Autodesk Inventor part; units mm, degrees
ref_plane "YZ Plane" through (0, 0, 0) normal (1, 0, 0) x (0, 1, 0)
ref_plane "XZ Plane" through (0, 0, 0) normal (0, 1, 0) x (-1, 0, 0)
ref_plane "XY Plane" through (0, 0, 0) normal (0, 0, 1) x (1, 0, 0)
sketch "Sketch1" plane through (0, 0, 0) normal (0, 0, 1) x (1, 0, 0)
  line L0 (0, 0) -> (90, 0)
  line L1 (90, 0) -> (90, -160)
  line L2 (90, -160) -> (0, -160)
  line L3 (0, -160) -> (0, 0)
  dimension "d0" = 90
  dimension "d1" = 160
extrude "Extrusion1" add sketch "Sketch1" along normal blind 1.6
sketch "Sketch2" plane through (0, 0, 1.6) normal (0, 0, 1) x (1, 0, 0)
  line L0 (5, -5) -> (85, -5)
  line L1 (85, -5) -> (85, -15)
  line L2 (85, -15) -> (5, -15)
  line L3 (5, -15) -> (5, -5)
  line L4 (90, 0) -> (0, 0)
  line L5 (0, 0) -> (0, -160)
  line L6 (90, -160) -> (90, 0)
  line L7 (5, -5) -> (15, -5)
  line L8 (15, -5) -> (15, -155)
  line L9 (15, -155) -> (5, -155)
  line L10 (5, -155) -> (5, -5)
  line L11 (0, -160) -> (90, -160)
  line L12 (5, -155) -> (85, -155)
  line L13 (85, -155) -> (85, -145)
  line L14 (85, -145) -> (5, -145)
  line L15 (5, -145) -> (5, -155)
  line L16 (85, -5) -> (75, -5)
  line L17 (75, -5) -> (75, -155)
  line L18 (75, -155) -> (85, -155)
  line L19 (85, -155) -> (85, -5)
  line L20 (5, -75) -> (85, -75)
  line L21 (85, -75) -> (85, -85)
  line L22 (85, -85) -> (5, -85)
  line L23 (5, -85) -> (5, -75)
  dimension "d4" = 5
  dimension "d5" = 5
  dimension "d6" = 5
  dimension "d7" = 10
  dimension "d8" = 10
  dimension "d9" = 5
  dimension "d10" = 80
  dimension "d11" = 10
  dimension "d12" = 10
  dimension "d13" = 80
  dimension "d14" = 10
  dimension "d15" = 75
extrude "Extrusion2" add sketch "Sketch2" along normal blind 4.6 contours L0 L8 L2 L3 | L0 L17 L2 L8 | L2 L8 L20 L10 | L0 L1 L2 L17 | L20 L8 L22 L10 | L2 L19 L20 L17 | L20 L17 L22 L8 | L22 L8 L14 L10 | L20 L19 L22 L17 | L14 L8 L9 L10 | L22 L19 L14 L17 | L14 L17 L12 L8 | L14 L13 L12 L17
sketch "Sketch3" plane through (0, 0, 6.2) normal (0, 0, 1) x (1, 0, 0)
  circle A0 centre (20, -10) radius 2.6
  circle A1 centre (53.3333, -10) radius 2.6
  circle A2 centre (36.6667, -10) radius 2.6
  circle A3 centre (80, -140) radius 2.6
  circle A4 centre (80, -123.3333) radius 2.6
  circle A5 centre (80, -107) radius 2.6
  circle A6 centre (80, -90) radius 2.6
  circle A7 centre (70, -150) radius 2.6
  circle A8 centre (53.3333, -150) radius 2.6
  circle A9 centre (36.6667, -150) radius 2.6
  circle A10 centre (20, -150) radius 2.6
  circle A11 centre (10, -140) radius 2.6
  circle A12 centre (10, -123.3333) radius 2.6
  circle A13 centre (10, -106.6667) radius 2.6
  circle A14 centre (10, -90) radius 2.6
  circle A15 centre (70, -80) radius 2.6
  circle A16 centre (53.3333, -80) radius 2.6
  circle A17 centre (36.6667, -80) radius 2.6
  circle A18 centre (20, -80) radius 2.6
  circle A19 centre (80, -70) radius 2.6
  circle A20 centre (80, -53.3333) radius 2.6
  circle A21 centre (80, -36.6667) radius 2.6
  circle A22 centre (80, -20) radius 2.6
  circle A23 centre (10, -70) radius 2.6
  circle A24 centre (10, -53.3333) radius 2.6
  circle A25 centre (10, -36.6667) radius 2.6
  circle A26 centre (10, -20) radius 2.6
  circle A27 centre (70, -10) radius 2.6
  line L0 (85, -155) -> (5, -155)
  line L1 (85, -5) -> (5, -5)
  line L2 (5, -5) -> (5, -155)
  line L3 (15, -75) -> (15, -15)
  line L4 (75, -15) -> (75, -75)
  line L5 (15, -15) -> (75, -15)
  line L6 (85, -155) -> (85, -5)
  line L7 (15, -85) -> (75, -85)
  line L8 (15, -145) -> (15, -85)
  point P0 (0, 0)
  point P1 (90, -155)
  dimension "d18" = 5.2
  dimension "d20" = 5.2
  dimension "d21" = 5.2
  dimension "d22" = 5.2
  dimension "d23" = 5.2
  dimension "d24" = 5.2
  dimension "d25" = 5.2
  dimension "d26" = 5.2
  dimension "d27" = 5.2
  dimension "d28" = 5.2
  dimension "d29" = 5.2
  dimension "d30" = 5.2
  dimension "d31" = 5.2
  dimension "d32" = 5.2
  dimension "d33" = 5.2
  dimension "d34" = 5.2
  dimension "d35" = 5.2
  dimension "d36" = 5.2
  dimension "d37" = 5.2
  dimension "d38" = 5.2
  dimension "d39" = 5.2
  dimension "d40" = 5.2
  dimension "d41" = 5.2
  dimension "d42" = 5.2
  dimension "d43" = 5.2
  dimension "d44" = 5.2
  dimension "d45" = 5.2
  dimension "d47" = 5.2
  dimension "d48" = 5
  dimension "d49" = 5
  dimension "d50" = 5
  dimension "d51" = 5
  dimension "d52" = 5
  dimension "d53" = 5
  dimension "d55" = 5
  dimension "d56" = 16.6667
  dimension "d57" = 16.6667
  dimension "d58" = 5
  dimension "d59" = 16.6667
  dimension "d60" = 16.6667
  dimension "d61" = 16.6667
  dimension "d62" = 5
  dimension "d63" = 5
  dimension "d64" = 5
  dimension "d65" = 16.6667
  dimension "d66" = 16.6667
  dimension "d67" = 16.6667
  dimension "d68" = 5
  dimension "d73" = 16.6667
  dimension "d74" = 16.6667
  dimension "d75" = 16.6667
extrude "Extrusion3" cut sketch "Sketch3" against normal through all contours A0 | A1 | A2 | A3 | A4 | A5 | A6 | A7 | A8 | A9 | A10 | A11 | A12 | A13 | A14 | A15 | A16 | A17 | A18 | A19 | A20 | A21 | A22 | A23 | A24 | A25 | A26 | A27
sketch "Sketch4" plane through (0, 0, 1.6) normal (0, 0, 1) x (1, 0, 0)
  line L0 (75, -15) -> (15, -15)
  line L1 (15, -15) -> (15, -75)
  line L2 (15, -75) -> (75, -75)
  line L3 (75, -75) -> (75, -15)
  line L4 (75, -85) -> (15, -85)
  line L5 (15, -85) -> (15, -145)
  line L6 (15, -145) -> (75, -145)
  line L7 (75, -145) -> (75, -85)
  line L8 (0, 0) -> (5, 0)
  line L9 (5, 0) -> (5, -155)
  line L10 (5, -155) -> (0, -155)
  line L11 (0, -155) -> (0, 0)
  line L12 (5, 0) -> (85, 0)
  line L13 (85, 0) -> (85, -5)
  line L14 (85, -5) -> (5, -5)
  line L15 (5, -5) -> (5, 0)
  line L16 (90, 0) -> (85, 0)
  line L17 (85, 0) -> (85, -155)
  line L18 (85, -155) -> (90, -155)
  line L19 (90, -155) -> (90, 0)
  line L20 (90, -160) -> (0, -160)
  line L21 (0, -155) -> (5, -155)
  line L22 (5, -155) -> (5, -160)
  line L23 (5, -160) -> (0, -160)
  line L24 (0, -160) -> (0, -155)
  line L25 (85, -155) -> (90, -155)
  line L26 (90, -155) -> (90, -160)
  line L27 (90, -160) -> (85, -160)
  line L28 (85, -160) -> (85, -155)
extrude "Extrusion4" cut sketch "Sketch4" against normal through all contours L3 L2 L1 L0 | L7 L6 L5 L4 | L8 L9 L10 L11 | L12 L13 L14 L9 | L10 L22 L20 L24 | L16 L19 L18 L17 L13 | L18 L26 L20 L28
fillet "Fillet1" radius 15 2 edges at (5, -5, 3.1) (85, -5, 3.1)
properties part number "large edition 3 open"
Could you check a few things on this model? Use its own coordinates, in mm. Give positions to 0.01 mm unless a question says otherwise; leave off trailing zeros. Loops run counter-clockwise (first coordinate to the right, second up) from the corner with the lowest first, then second, coordinate; pieces in that order, holes last. Notation, with made-up numbers: (52.5, 14) - (81.5, 14) arc R20 ccw to (81.5, 26) - close; hole circle Ø5 at (-2, 13). An arc over 180 degrees is marked (long way). Use one line per item in the form item = value.
1. I want a section at B-B (y = -119). Please give me the cut outline in (x, z).
Response values:
outline = (5, 0) - (15, 0) - (15, 6.2) - (5, 6.2) - close; (75, 0) - (85, 0) - (85, 6.2) - (75, 6.2) - close
2. I want a section at D-D (x = 79.5). Give the number of separate pieces and of enclosed holes in the cut face, and give its area (3 significant figures).
Response values:
separate_pieces = 9
enclosed_holes = 0
area = 664 mm²
3. Thinking about a two-plate mould opening in X: for faces 1 (the face through (37.866, -12.307, 3.143)), 2 (the face through (85, -89, 3)), 3 (the face through (9.662, -50.755, 3.143)), 4 (the face through (5, -89, 3)), which applies, released by +X, released by -X, zero draft, split by the parting line, or undercut?
Response values:
face_1 = undercut
face_2 = released by +X
face_3 = undercut
face_4 = released by -X
4. I'm going to push a flat-ended pin straight in: pin 1 Ø3 at (x, z) = (47.5, 4.5) entering from -Y. Where does the tip first touch, or does it pass through?
Response values:
pin_1 = -155
5. I want a section at A-A (y = -80). Please give me the cut outline in (x, z).
Response values:
outline = (5, 0) - (17.4, 0) - (17.4, 6.2) - (5, 6.2) - close; (22.6, 0) - (34.07, 0) - (34.07, 6.2) - (22.6, 6.2) - close; (39.27, 0) - (50.73, 0) - (50.73, 6.2) - (39.27, 6.2) - close; (55.93, 0) - (67.4, 0) - (67.4, 6.2) - (55.93, 6.2) - close; (72.6, 0) - (85, 0) - (85, 6.2) - (72.6, 6.2) - close
6. I need wall thicknesses on probe 1 along Y at (x, z) = (63.5, 3.75); probe 2 along Y at (x, z) = (25.5, 0.5); probe 3 along X at (y, z) = (-150, 2.25). Which ranges of each line are inside material? Lowest first, please.
Response values:
probe_1 = -155 to -145, -85 to -75, -15 to -5
probe_2 = -160 to -145, -85 to -75, -15 to -5
probe_3 = 5 to 17.4, 22.6 to 34.07, 39.27 to 50.73, 55.93 to 67.4, 72.6 to 85
7. I want a section at C-C (x = 30). Please give me the cut outline in (y, z), and give its area (3 significant figures).
Response values:
outline = (-160, 0) - (-145, 0) - (-145, 6.2) - (-155, 6.2) - (-155, 1.6) - (-160, 1.6) - close; (-85, 0) - (-75, 0) - (-75, 6.2) - (-85, 6.2) - close; (-15, 0) - (-5, 0) - (-5, 6.2) - (-15, 6.2) - close
area = 194 mm²
